Can you work these out from the model? Positions are in its coordinate system, mm. Face numbers are marked on the shaded views. A direction names the side the tool comes from. Give positions to 0.01 mm unless a question says otherwise; leave off trailing zeros. Order: outer loops, then holes, each group sorted by start corner. A loop starts at its lowest first (then second) coordinate and runs counter-clockwise, first axis right, second up. Notation, with made-up numbers: (74, 22.25) - (101, 22.25) arc R32 ccw to (101, 61.25) - close; hole circle Ø2 at (-39.5, 58.25). An arc over 180 degrees is marked (long way). Write each question's results on one line, items separated by ' | '. Start each with the question number.
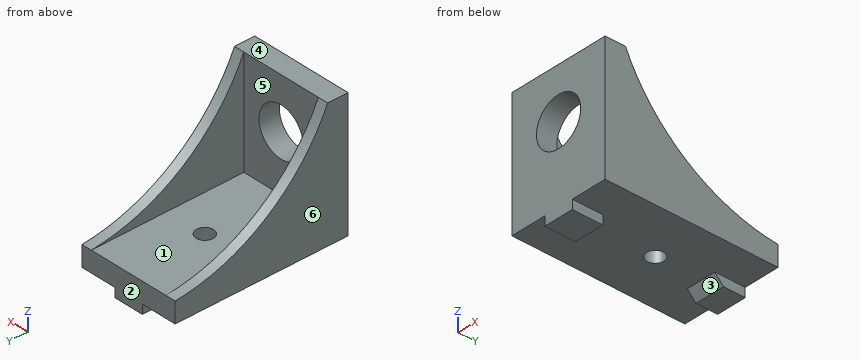
from build123d import *

# Parameters (mm, degrees)
SKETCH090_W     = 20
SKETCH090_H     = 30
SKETCH090_R     = 1.7
PAD021_DEPTH    = 4
SKETCH091_W     = 20
SKETCH091_H     = 25
SKETCH091_R     = 4.75
PAD022_DEPTH    = 4
PAD023_DEPTH    = 2
PAD024_DEPTH    = 2
SKETCH094_W     = 5.9
SKETCH094_H     = 6
PAD025_DEPTH    = 1.8
CHAMFER051_SIZE = 1.75


with BuildPart() as part:
    # Sketch090 → Pad021 (new body)
    with BuildSketch(Plane.XY):
        Rectangle(SKETCH090_W, SKETCH090_H)
        Circle(SKETCH090_R, mode=Mode.SUBTRACT)
    extrude(amount=PAD021_DEPTH)

    # Sketch091 → Pad022 (join)
    with BuildSketch(Plane.XZ.offset(15)):
        with Locations((0, 12.5)):
            Rectangle(SKETCH091_W, SKETCH091_H)
        with Locations((0, 15)):
            Circle(SKETCH091_R, mode=Mode.SUBTRACT)
    extrude(amount=PAD022_DEPTH)

    # Sketch092 → Pad023 (join)
    with BuildSketch(Plane.YZ.offset(8)):
        with BuildLine():
            Line((-15, 25), (-15, 4))
            Line((-15, 4), (15, 4))
            ThreePointArc((-15, 25), (-2.8696242204, 10.400536828), (15, 4))
        make_face()
    extrude(amount=PAD023_DEPTH)

    # Sketch093 → Pad024 (join)
    with BuildSketch(Plane.YZ.offset(-8)):
        with BuildLine():
            Line((-15, 25), (-15, 4))
            Line((-15, 4), (15, 4))
            ThreePointArc((-15, 25), (-2.8696242204, 10.400536828), (15, 4))
        make_face()
    extrude(amount=-PAD024_DEPTH)

    # Sketch094 (on Face4 of Pad024) → Pad025 (join)
    with BuildSketch(Plane(origin=(0, 0, 0), x_dir=(1, 0, 0), z_dir=(0, 0, -1))):
        with Locations((0, 16)):
            Rectangle(SKETCH094_W, SKETCH094_H)
        with Locations((0, -12)):
            Rectangle(SKETCH094_W, SKETCH094_H)
    extrude(amount=PAD025_DEPTH)

    # Chamfer051
    chamfer051_edges = [part.edges().sort_by_distance(p)[0] for p in [
        (0, 9, -1.8),
    ]]
    chamfer(chamfer051_edges, length=CHAMFER051_SIZE)


solid = part.part
Q1. If I drill on probe 1 along Y at (x, z) = (0, 1.6); probe 2 along X at (y, z) = (-9.5, 4.25); probe 3 along Y at (x, z) = (4.75, 9.25), over which ranges is the centre line in solid material (lowest first)? Write a range as from..to.
Q2. Will these pins go through, and if not, where does the flat tip stop? P1, Ø2, axis at x = -2, y = -5.5, coming from the +Z side; P2, Ø1, axis at x = -5.5, z = 13.5, coming from the +Y side; P3, Ø1.4, axis at y = 12, z = -1, coming from the -X side.
Q3. If we section it at B-B (z = 15): Please give me the cut outline in (x, y).
Q4. If we section it at C-C (x = 0): Please give me the cut outline in (y, z).
Q5. If we section it at D-D (x = 5.5): Please give me the cut outline in (y, z).
Q6. If we section it at A-A (x = -2.25): Please give me the cut outline in (y, z), plus the area to 3 significant figures.
Q7. Thinking about a two-plate mould opening in X: for the marked faces 4, 5 and 6, which applies, released by +X, released by -X, zero draft, split by the parting line, or undercut?
Q8. Which directions (+Z, -Z, +X, -X, +Y, -Y) give clear straight access to the entire face, cutting with the end or side of a thin tool? Please do the marked faces 1, 2 and 3.
Findings below:
1) probe 1: y = -19..-1.7, 1.7..15 | probe 2: x = -10..-8, 8..10 | probe 3: y = -19..-15
2) P1: stops at z = 4 | P2: stops at y = -15 | P3: stops at x = -2.95
3) outline: (-10, -19) - (-4.75, -19) - (-4.75, -15) - (-8, -15) - (-8, -8.23) - (-10, -8.23) - close; (4.75, -19) - (10, -19) - (10, -8.23) - (8, -8.23) - (8, -15) - (4.75, -15) - close
4) outline: (-19, -1.8) - (-13, -1.8) - (-13, 0) - (-1.7, 0) - (-1.7, 4) - (-15, 4) - (-15, 10.25) - (-19, 10.25) - close; (-19, 19.75) - (-15, 19.75) - (-15, 25) - (-19, 25) - close; (1.7, 0) - (9, 0) - (9, -0.05) - (10.75, -1.8) - (15, -1.8) - (15, 4) - (1.7, 4) - close
5) outline: (-19, 0) - (15, 0) - (15, 4) - (-15, 4) - (-15, 25) - (-19, 25) - close
6) outline: (-19, -1.8) - (-13, -1.8) - (-13, 0) - (9, 0) - (9, -0.05) - (10.75, -1.8) - (15, -1.8) - (15, 4) - (-15, 4) - (-15, 10.82) - (-19, 10.82) - close; (-19, 19.18) - (-15, 19.18) - (-15, 25) - (-19, 25) - close | area: 207 mm2
7) face 4: zero draft | face 5: undercut | face 6: released by -X
8) face 1: +Z, +Y | face 2: +Z, -Z, +X, -X, +Y | face 3: -Z, +X, -X
